Design review of the part built by this model. Coordinates are the model's own, in mm. Face numbers are marked on the shaded views. A direction names the side the tool comes from. Round coordinates to 2 decimals unless told otherwise and drop trailing zeros. Write each loop counter-clockwise with the first axis right and the second up, starting at its lowest first coordinate (ties: lowest second). Pieces come first, ordered by that corner, then holes.
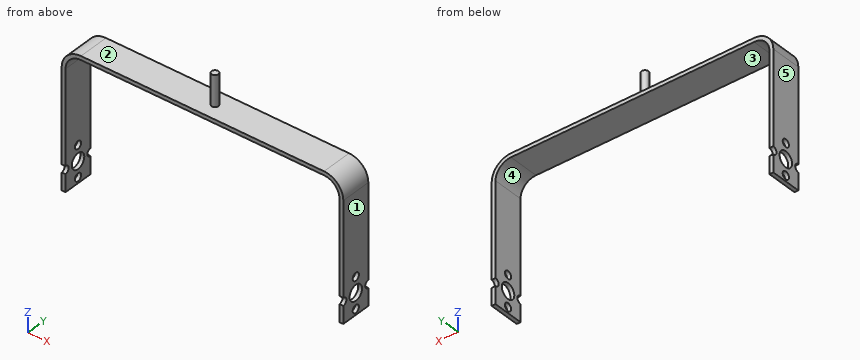
from build123d import *

# Parameters (mm, degrees)
BOSS_EXTRUDE1_DEPTH = 16
FILLET1_R           = 8
FILLET2_R           = 10
SKETCH2_R           = 4
SKETCH2_R_2         = 2
CUT_EXTRUDE1_DEPTH  = 147.05
SKETCH3_R           = 1.75
BOSS_EXTRUDE2_DEPTH = 15.875


with BuildPart() as part:
    # Sketch1 → Boss-Extrude1 (new body)
    with BuildSketch(Plane(origin=(0, 0, 0), x_dir=(1, 0, 0), z_dir=(0, 1, 0))):
        Polygon((0, 0), (142.05, 0), (142.05, 69.325), (144.05, 69.325), (144.05, -2), (-2, -2), (-2, 69.325), (0, 69.325), align=None)
    extrude(amount=BOSS_EXTRUDE1_DEPTH)

    # Fillet1
    fillet1_edges = [part.edges().sort_by_distance(p)[0] for p in [
        (0, 8, 0),
        (142.05, 8, 0),
    ]]
    fillet(fillet1_edges, radius=FILLET1_R)

    # Fillet2
    fillet2_edges = [part.edges().sort_by_distance(p)[0] for p in [
        (144.05, 8, 2),
        (-2, 8, 2),
    ]]
    fillet(fillet2_edges, radius=FILLET2_R)

    # Sketch2 → Cut-Extrude1 (cut, through all)
    with BuildSketch(Plane(origin=(144.05, 0, 0), x_dir=(0, 0, -1), z_dir=(1, 0, 0))):
        with Locations((58.325, 8)):
            Circle(SKETCH2_R)
        with Locations((66.325, 8)):
            Circle(SKETCH2_R_2)
        with Locations((58.325, 0)):
            Circle(SKETCH2_R_2)
        with Locations((50.325, 8)):
            Circle(SKETCH2_R_2)
        with Locations((58.325, 16)):
            Circle(SKETCH2_R_2)
    extrude(amount=-CUT_EXTRUDE1_DEPTH, mode=Mode.SUBTRACT)

    # Sketch3 → Boss-Extrude2 (add)
    with BuildSketch(Plane.XY.offset(2)):
        with Locations((71.025, 8)):
            Circle(SKETCH3_R)
    extrude(amount=BOSS_EXTRUDE2_DEPTH)


solid = part.part
1) Add section B-B on y = 8. Count the separate pieces of the cut face and the enclosed holes in it, and give its area (3 significant figures).
2) Add section C-C on x = 107. State the section outline as (y, z) points, and give its area (3 significant figures).
3) For the marked faces 4 and 5, list the 3-axis set-ups (+Z, -Z, +X, -X, +Y, -Y) from which the entire face can be reached by the end or side of a thin tool; tool diameter is ignored.
4) The part is to be moulded in two halves that separate along X. For the marked faces 1, 2 and 3, say which applies: pulls with the +X half, pulls with the -X half, needs draft (parallel to the pull), parting line crosses it, or undercut.
5) For P1, Ø5, axis at x = 41, y = 5, coming from the -Z side; P2, Ø6, axis at x = 20.5, y = 11, coming from the +Z side; P3, Ø8, axis at y = 14, z = -1.5, coming from the -X side, all flat-tipped, find the tip position at first contact; note any pin that passes through.
6) Add section A-A on z = -20.5. State the section outline as (x, y) points, and give its area (3 significant figures).
7) For line 1 along X through (y, z) = (12, -18.5); line 2 along Z through (x, y) = (122.5, 2.75); line 3 along X through (y, z) = (0.5, -1), list the stretches that pass through material, from the lowest coordinate up.
Computed:
1. separate pieces: 7
1. enclosed holes: 0
1. area: 546 mm2
2. outline: (0, 0) - (16, 0) - (16, 2) - (0, 2) - close
2. area: 32.0 mm2
3. face 4: -Z, +Y, -Y
3. face 5: +Z, -Z, -X, +Y, -Y
4. face 1: pulls with the +X half
4. face 2: needs draft
4. face 3: undercut
5. P1: stops at z = 0
5. P2: stops at z = 2
5. P3: stops at x = -1.68
6. outline: (-2, 0) - (0, 0) - (0, 16) - (-2, 16) - close; (142.05, 0) - (144.05, 0) - (144.05, 16) - (142.05, 16) - close
6. area: 64.0 mm2
7. line 1: x = -2 to 0, 142.05 to 144.05
7. line 2: z = 0 to 2
7. line 3: x = 0.86 to 4.13, 137.92 to 141.19
